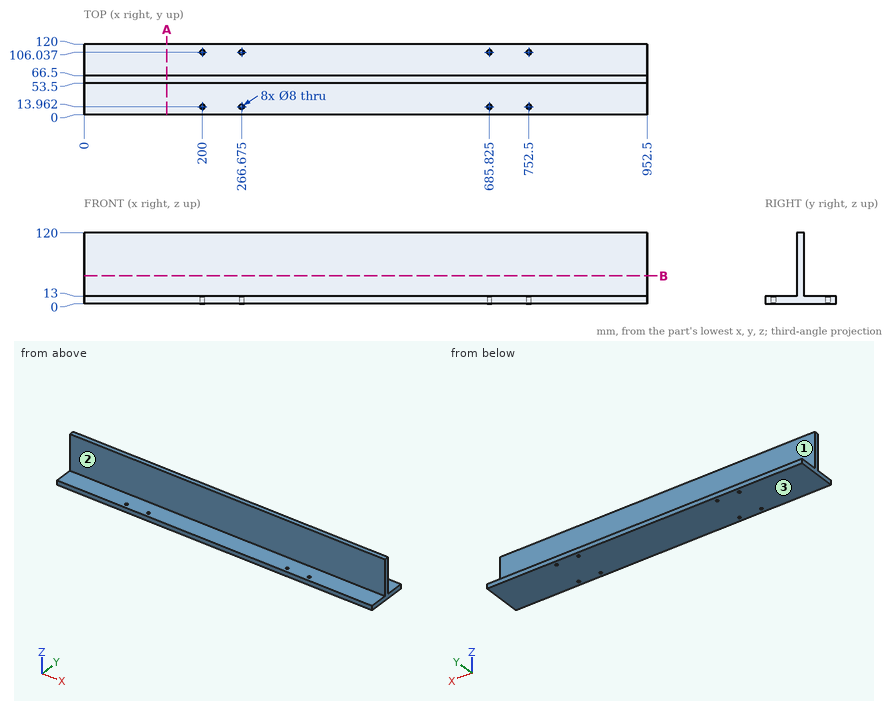
For this review, use the dimensioned drawing (mm, ordinates from the lowest corner) and the shaded views. A direction names the side the tool comes from. Round coordinates to 2 decimals unless told otherwise and drop trailing zeros. Order: outer loops, then holes, each group sorted by start corner. A loop starts at its lowest first (then second) coordinate and runs counter-clockwise, first axis right, second up. Notation, with made-up numbers: (-6, 64) -> (36, 64) arc R30 cw to (36, 103) -> close; hole circle Ø1 at (2.25, 7). An arc over 180 degrees is marked (long way). Use CSV: the item, a comma, the result in double quotes. Start each with the question number.
(1) Consider section A-A on x = 140. Write out the cut boundary in (y, z), and give its area (3 significant figures).
(2) Consider section B-B on z = 47.5. Write out the cut boundary in (x, y).
(3) Tool access review of the marked faces 1, 2 and 3: name each direction out of +Z, -Z, +X, -X, +Y, -Y from which nothing blocks a thin tool from reaching the whole face with its end or side.
(4) Wall thickness on probe 1 along Y at (x, z) = (752, 6) (1 decimal); probe 2 along Y at (x, z) = (200, 4.5); probe 3 along Y at (x, z) = (870, 88.5): over which ranges is each line inside the solid? List them lowest first. Write a range as from..to.
(5) Insertion check: pin 1 (2 mm diameter, centred on x = 480, z = 40.5, fed in from +Y); pin 2 (7 mm diameter, centred on x = 200, y = 106.04, fed in from +Z); pin 3 (10 mm diameter, centred on x = 306.5, z = 56.5, fed in from -Y); pin 4 (9 mm diameter, centred on x = 685.82, y = 13.96, fed in from +Z). Each pin has a flat end and moves straight along its axis. Give the tip position at first contact, or say it passes through.
Responses:
1,outline,"(0, 0) -> (120, 0) -> (120, 13) -> (66.5, 13) -> (66.5, 120) -> (53.5, 120) -> (53.5, 13) -> (0, 13) -> close"
1,area,"2,950 mm²"
2,outline,"(0, 53.5) -> (952.5, 53.5) -> (952.5, 66.5) -> (0, 66.5) -> close"
3,face 1,"+Z, +X, -X, +Y"
3,face 2,"+Z, +X, -X, -Y"
3,face 3,"-Z, +X, -X, +Y, -Y"
4,probe 1,"0..10, 17.9..102.1, 110..120"
4,probe 2,"0..9.96, 17.96..102.04, 110.04..120"
4,probe 3,"53.5..66.5"
5,pin 1,"y = 66.5"
5,pin 2,"through"
5,pin 3,"y = 53.5"
5,pin 4,"z = 13"
